The listing builds one solid part. Answer for the finished solid, in the listing's coordinates (mm). Round coordinates to 2 decimals unless told otherwise and drop trailing zeros. Write each loop counter-clockwise with the first axis right and the second up, starting at its lowest first coordinate (ties: lowest second). Pieces come first, ordered by that corner, then holes.
(1) A cutting plane is placed at A-A, the plane y = 3.9. Give the number of separate pieces and of enclosed holes in the cut face, and give its area (3 significant figures).
(2) Find the intervals of material crossed by probe 1 along X at (y, z) = (1.2, 90); probe 2 along Z at (x, y) = (-147.5, 4); probe 3 along X at (y, z) = (3.6, 49), in increasing order.
(3) A cutting plane is placed at B-B, the plane x = -164.5. Give the vertices of the cut face in (y, z).
(4) Each of these flat-tipped pins is pushed along its axis until it touches: pin 1 Ø2.5 at (y, z) = (3.5, 81.5) entering from -X; pin 2 Ø1.5 at (x, y) = (-149.5, 2.5) entering from +Z. Where does it stop, or does it pass through?
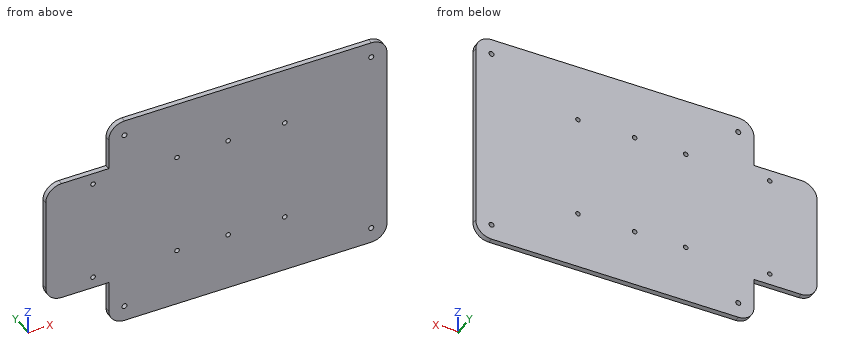
from build123d import *

# Parameters (mm, degrees)
SKETCH_1_W          = 265
SKETCH_1_H          = 210
EXTRUDE_1_DEPTH     = 5
SKETCH_3_R          = 2.4
CUT_EXTRUDE_1_DEPTH = 5
FILLET_1_R          = 15
SKETCH_4_W          = 60
SKETCH_4_H          = 120
EXTRUDE_3_DEPTH     = 5
FILLET_2_R          = 15
SKETCH_6_R          = 2.2
CUT_EXTRUDE_2_DEPTH = 24
SKETCH_7_R          = 2.2
CUT_EXTRUDE_3_DEPTH = 10


with BuildPart() as part:
    # 草图1 → 凸台-拉伸1 (new body)
    with BuildSketch(Plane(origin=(0, 0, 0), x_dir=(1, 0, 0), z_dir=(0, 1, 0))):
        Rectangle(SKETCH_1_W, SKETCH_1_H)
    extrude(amount=EXTRUDE_1_DEPTH)

    # 草图3 → 切除-拉伸1 (cut)
    with BuildSketch(Plane(origin=(0, 5, 0), x_dir=(1, 0, 0), z_dir=(0, 1, 0))):
        with Locations(Location((-117.5, 90, 0), (0, 0, 270))):
            Circle(SKETCH_3_R)
        with Locations(Location((117.5, 90, 0), (0, 0, 90))):
            Circle(SKETCH_3_R)
        with Locations(Location((117.5, -90, 0), (0, 0, 270))):
            Circle(SKETCH_3_R)
        with Locations(Location((-117.5, -90, 0), (0, 0, 90))):
            Circle(SKETCH_3_R)
    extrude(amount=-CUT_EXTRUDE_1_DEPTH, mode=Mode.SUBTRACT)

    # 圆角1
    fillet_1_edges = [part.edges().sort_by_distance(p)[0] for p in [
        (-132.5, 2.5, -105),
        (132.5, 2.5, -105),
        (132.5, 2.5, 105),
        (-132.5, 2.5, 105),
    ]]
    fillet(fillet_1_edges, radius=FILLET_1_R)

    # 草图4 → 凸台-拉伸3 (add)
    with BuildSketch(Plane(origin=(0, 0, 0), x_dir=(1, 0, 0), z_dir=(0, 1, 0))):
        with Locations((-162.5, 0)):
            Rectangle(SKETCH_4_W, SKETCH_4_H)
    extrude(amount=EXTRUDE_3_DEPTH)

    # 圆角2
    fillet_2_edges = [part.edges().sort_by_distance(p)[0] for p in [
        (-192.5, 2.5, -60),
        (-192.5, 2.5, 60),
    ]]
    fillet(fillet_2_edges, radius=FILLET_2_R)

    # 草图6 → 切除-拉伸2 (cut)
    with BuildSketch(Plane(origin=(0, 5, 0), x_dir=(1, 0, 0), z_dir=(0, 1, 0))):
        with Locations(Location((-147.5, 49, 0), (0, 0, 270))):
            Circle(SKETCH_6_R)
        with Locations(Location((-67.5, 49, 0), (0, 0, 270))):
            Circle(SKETCH_6_R)
        with Locations(Location((-67.5, -49, 0), (0, 0, 270))):
            Circle(SKETCH_6_R)
        with Locations(Location((-147.5, -49, 0), (0, 0, 270))):
            Circle(SKETCH_6_R)
    extrude(amount=-CUT_EXTRUDE_2_DEPTH, mode=Mode.SUBTRACT)

    # 草图7 → 切除-拉伸3 (cut)
    with BuildSketch(Plane(origin=(0, 5, 0), x_dir=(1, 0, 0), z_dir=(0, 1, 0))):
        with Locations(Location((-18.8, 49.5, 0), (0, 0, 270))):
            Circle(SKETCH_7_R)
        with Locations(Location((35.2, 49.5, 0), (0, 0, 270))):
            Circle(SKETCH_7_R)
        with Locations(Location((35.2, -49.5, 0), (0, 0, 270))):
            Circle(SKETCH_7_R)
        with Locations(Location((-18.8, -49.5, 0), (0, 0, 270))):
            Circle(SKETCH_7_R)
    extrude(amount=-CUT_EXTRUDE_3_DEPTH, mode=Mode.SUBTRACT)


solid = part.part
Solutions:
1. separate pieces: 1
1. enclosed holes: 12
1. area: 62,400 mm2
2. probe 1: x = -132.5 to -119.9, -115.1 to 115.1, 119.9 to 132.5
2. probe 2: z = -60 to -51.2, -46.8 to 46.8, 51.2 to 60
2. probe 3: x = -191.96 to -149.7, -145.3 to -69.7, -65.3 to -20.94, -16.66 to 33.06, 37.34 to 132.5
3. outline: (0, -60) - (5, -60) - (5, 60) - (0, 60) - close
4. pin 1: stops at x = -132.5
4. pin 2: stops at z = 60
